```python
from build123d import *

# Parameters (mm, degrees)
SKETCH2_W            = 113
SKETCH2_H            = 57
BOSS_EXTRUDE1_DEPTH  = 57
SKETCH11_R           = 5
BOSS_EXTRUDE12_DEPTH = 24
SKETCH11_6_R         = 19
SKETCH11_6_R_2       = 5
BOSS_EXTRUDE13_DEPTH = 1.6
SKETCH13_R           = 2
CUT_EXTRUDE1_DEPTH   = 113
CUT_EXTRUDE4_START   = -20
CUT_EXTRUDE4_DEPTH   = 20
CUT_EXTRUDE5_START   = -108
SKETCH22_R           = 2
CUT_EXTRUDE5_DEPTH   = 108
FILLET1_R            = 2
FILLET2_R            = 2


with BuildPart() as part:
    # Sketch2 → Boss-Extrude1 (new body)
    with BuildSketch(Plane(origin=(0, 0, 0), x_dir=(1, 0, 0), z_dir=(0, 1, 0))):
        with Locations((56.5, 28.5)):
            Rectangle(SKETCH2_W, SKETCH2_H)
    extrude(amount=BOSS_EXTRUDE1_DEPTH)

    # Sketch11 → Boss-Extrude12 (add)
    with BuildSketch(Plane.ZY):
        with Locations(Location((-28.5, 28.5, 0), (0, 0, 180))):
            Circle(SKETCH11_R)
    extrude(amount=BOSS_EXTRUDE12_DEPTH)

    # Sketch11_6 → Boss-Extrude13 (add)
    with BuildSketch(Plane.ZY):
        with Locations(Location((-28.5, 28.5, 0), (0, 0, 180))):
            Circle(SKETCH11_6_R)
        with Locations((-28.5, 28.5)):
            Circle(SKETCH11_6_R_2, mode=Mode.SUBTRACT)
    extrude(amount=BOSS_EXTRUDE13_DEPTH)

    # Sketch13 → Cut-Extrude1 (cut)
    with BuildSketch(Plane.ZY):
        with Locations((-5, 5)):
            Circle(SKETCH13_R)
        with Locations((-52, 5)):
            Circle(SKETCH13_R)
        with Locations((-52, 52)):
            Circle(SKETCH13_R)
        with Locations((-5, 52)):
            Circle(SKETCH13_R)
    extrude(amount=-CUT_EXTRUDE1_DEPTH, mode=Mode.SUBTRACT)

    # Sketch14 → Cut-Extrude4 (cut)
    with BuildSketch(Plane.ZY.offset(24).offset(CUT_EXTRUDE4_START)):
        with BuildLine():
            Line((-28.5, 24.207845288), (-31.06464577, 24.207845288))
            ThreePointArc((-31.06464577, 24.207845288), (-28.5, 23.5), (-25.93535423, 24.207845288))
            Line((-25.93535423, 24.207845288), (-28.5, 24.207845288))
        make_face()
    extrude(amount=CUT_EXTRUDE4_DEPTH, mode=Mode.SUBTRACT)

    # Sketch22 → Cut-Extrude5 (cut)
    # profile 1 of 4: a face of its own
    with BuildSketch(Plane(origin=(113, 0, 0), x_dir=(0, 0, -1), z_dir=(1, 0, 0)).offset(CUT_EXTRUDE5_START)):
        with BuildLine():
            ThreePointArc((47.5, 52), (48.818019485, 48.818019485), (52, 47.5))
            Line((52, 47.5), (57, 47.5))
            Line((57, 47.5), (57, 57))
            Line((57, 57), (47.5, 57))
            Line((47.5, 57), (47.5, 52))
        make_face()
        with Locations(Location((52, 52, 0), (0, 0, 180))):
            Circle(SKETCH22_R, mode=Mode.SUBTRACT)
    # profile 2 of 4: a face of its own
    with BuildSketch(Plane(origin=(113, 0, 0), x_dir=(0, 0, -1), z_dir=(1, 0, 0)).offset(CUT_EXTRUDE5_START)):
        with BuildLine():
            Line((9.5, 52), (9.5, 57))
            Line((9.5, 57), (0, 57))
            Line((0, 57), (0, 47.5))
            Line((0, 47.5), (5, 47.5))
            ThreePointArc((5, 47.5), (8.181980515, 48.818019485), (9.5, 52))
        make_face()
        with Locations(Location((5, 52, 0), (0, 0, 180))):
            Circle(SKETCH22_R, mode=Mode.SUBTRACT)
    # profile 3 of 4: a face of its own
    with BuildSketch(Plane(origin=(113, 0, 0), x_dir=(0, 0, -1), z_dir=(1, 0, 0)).offset(CUT_EXTRUDE5_START)):
        with BuildLine():
            Line((57, 0), (57, 9.5))
            Line((57, 9.5), (52, 9.5))
            ThreePointArc((52, 9.5), (48.818019485, 8.181980515), (47.5, 5))
            Line((47.5, 5), (47.5, 0))
            Line((47.5, 0), (57, 0))
        make_face()
        with Locations(Location((52, 5, 0), (0, 0, 180))):
            Circle(SKETCH22_R, mode=Mode.SUBTRACT)
    # profile 4 of 4: a face of its own
    with BuildSketch(Plane(origin=(113, 0, 0), x_dir=(0, 0, -1), z_dir=(1, 0, 0)).offset(CUT_EXTRUDE5_START)):
        with BuildLine():
            Line((0, 0), (9.5, 0))
            Line((9.5, 0), (9.5, 5))
            ThreePointArc((9.5, 5), (8.181980515, 8.181980515), (5, 9.5))
            Line((5, 9.5), (0, 9.5))
            Line((0, 9.5), (0, 0))
        make_face()
        with Locations(Location((5, 5, 0), (0, 0, 180))):
            Circle(SKETCH22_R, mode=Mode.SUBTRACT)
    extrude(amount=CUT_EXTRUDE5_DEPTH, mode=Mode.SUBTRACT)

    # Fillet1
    fillet1_edges = [part.edges().sort_by_distance(p)[0] for p in [
        (59, 0, -9.5),
        (59, 9.5, 0),
        (59, 57, -47.5),
        (59, 47.5, -57),
        (59, 47.5, 0),
        (59, 57, -9.5),
        (59, 9.5, -57),
        (59, 0, -47.5),
    ]]
    fillet(fillet1_edges, radius=FILLET1_R)

    # Fillet2
    fillet2_edges = [part.edges().sort_by_distance(p)[0] for p in [
        (2.5, 57, -57),
        (2.5, 0, 0),
        (2.5, 57, 0),
        (2.5, 0, -57),
    ]]
    fillet(fillet2_edges, radius=FILLET2_R)


solid = part.part
```
For this review, take the finished solid that the model builds, in its own axes (mm). A direction names the side the tool comes from. Give positions to 0.01 mm unless a question says otherwise; leave off trailing zeros. Write each loop counter-clockwise with the first axis right and the second up, starting at its lowest first coordinate (ties: lowest second). Pieces come first, ordered by that corner, then holes. Notation, with made-up numbers: M -33,0 L -21,0 A19 ccw -21,36 Z; hole C -16.5,51 d1. An arc over 180 degrees is marked long. Answer as a JSON object with one key per item and string values. Group by question number.
Item 1: Consider section A-A on z = -28.5. Write out the cut boundary in (x, y).
Item 2: Consider section B-B on x = 74.5. Write out the cut boundary in (y, z).
Item 3: Consider section C-C on y = 22. Write out the cut boundary in (x, z).
Item 4: Tool access review of faces 5 (the cylindrical face through (58.244, 8.217, -48.853)), 6 (the cylindrical face through (-12.64, 33.38, -27.42)), 7 (the flat face through (58, 54, -47.5)), 8 (the cylindrical face through (58.244, 48.783, -8.147)): name each direction out of +Z, -Z, +X, -X, +Y, -Y from which nothing blocks a thin tool from reaching the whole face with its end or side.
Item 5: Consider section D-D on z = -42. Write out the cut boundary in (x, y), plus the area to 3 significant figures.
Item 6: For probe 1 along Z at (x, y) = (3, 5); probe 2 along Y at (x, z) = (1.6, -52); probe 3 along X at (y, z) = (54, -2), list the stretches that pass through material, from the lowest coordinate up. Write a range as [from, to].
Item 7: For pin 1 Ø3.5 at (y, z) = (5.5, -4.5) entering from +X; pin 2 Ø3.5 at (x, z) = (64.5, -54) entering from +Y; pin 3 Ø2.5 at (x, z) = (70, -4) entering from -Y, all flat-tipped, find the tip position at first contact; note any pin that passes through.
Item 8: Draft analysis for pull direction Y (two halves, no side actions). For faces 1 (the cylindrical face through (2.465, 50.226, -51.077)), 2 (the flat face through (58, 9.5, -54)), 3 (the flat face through (58, 4, -47.5)), 4 (the cylindrical face through (2.465, 50.226, -4.077)), state which applies: +Y half, -Y half, draft (parallel to the pull), parting line (faces both ways), or undercut.
Check result:
{
 "1": {"outline": "M -24,24.21 L -4,24.21 L -4,23.5 L -1.6,23.5 L -1.6,9.5 L 0,9.5 L 0,0 L 113,0 L 113,57 L 0,57 L 0,47.5 L -1.6,47.5 L -1.6,33.5 L -24,33.5 Z"},
 "2": {"outline": "M 0,-45.5 A2 ccw 2,-47.5 L 5,-47.5 A4.5 cw 9.5,-52 L 9.5,-55 A2 ccw 11.5,-57 L 45.5,-57 A2 ccw 47.5,-55 L 47.5,-52 A4.5 cw 52,-47.5 L 55,-47.5 A2 ccw 57,-45.5 L 57,-11.5 A2 ccw 55,-9.5 L 52,-9.5 A4.5 cw 47.5,-5 L 47.5,-2 A2 ccw 45.5,0 L 11.5,0 A2 ccw 9.5,-2 L 9.5,-5 A4.5 cw 5,-9.5 L 2,-9.5 A2 ccw 0,-11.5 Z"},
 "3": {"outline": "M -1.6,-46.35 L 0,-46.35 L 0,-57 L 113,-57 L 113,0 L 0,0 L 0,-10.65 L -1.6,-10.65 Z"},
 "4": {"face 5": "-Z, +X, -Y", "face 6": "-X", "face 7": "-Z, +X, +Y", "face 8": "+Z, +X, +Y"},
 "5": {"outline": "M -1.6,15.13 L 0,15.13 L 0,0 L 113,0 L 113,57 L 0,57 L 0,41.87 L -1.6,41.87 Z", "area": "6,480 mm^2"},
 "6": {"probe 1": "z = [-57, -54], [-50, -7], [-3, 0]", "probe 2": "y = [0, 3], [7, 50], [54, 57]", "probe 3": "x = [0, 5]"},
 "7": {"pin 1": "stops at x = 5", "pin 2": "stops at y = 47.5", "pin 3": "stops at y = 9.49"},
 "8": {"face 1": "undercut", "face 2": "-Y half", "face 3": "draft", "face 4": "undercut"}
}
